from build123d import *

# Parameters (mm, degrees)
F0_W     = 57.15
F0_H     = 31.75
F1_DEPTH = 25.4
F3_DEPTH = 25.4


with BuildPart() as f1:
    # F0 (on Front) → F1 (new body)
    with BuildSketch(Plane.XZ):
        with Locations((28.575, 15.875)):
            Rectangle(F0_W, F0_H)
    extrude(amount=F1_DEPTH)

    # F2 (on face) → F3 (cut)
    with BuildSketch(Plane.XZ.offset(25.4)):
        with BuildLine():
            Line((57.15, 31.75), (38.1, 31.75))
            ThreePointArc((38.1, 31.75), (43.6796158184, 18.2796158184), (57.15, 12.7))
            Line((57.15, 12.7), (57.15, 31.75))
        make_face()
        with BuildLine():
            ThreePointArc((0, 25.4), (2.5236444149, 29.2263555851), (6.35, 31.75))
            Line((6.35, 31.75), (0, 31.75))
            Line((0, 31.75), (0, 25.4))
        make_face()
    extrude(amount=-F3_DEPTH, mode=Mode.SUBTRACT)


solid = f1.part
Geometry check sheet. Reference: the model listing, model coordinates, mm. Round coordinates to 2 decimals unless told otherwise and drop trailing zeros. Order: outer loops, then holes, each group sorted by start corner. A loop starts at its lowest first (then second) coordinate and runs counter-clockwise, first axis right, second up. Notation, with made-up numbers: M 70.5,-37.75 L 82.5,-37.75 A17 ccw 82.5,-23.75 Z; hole C -34,-0.75 d4. An arc over 180 degrees is marked long. Answer in a Markdown table with one row per item. Add a question column.
Item 1: Sectioned sample at A-A, the plane y = -23.5. Enter the section's corners in (x, z).
Item 2: Sectioned sample at C-C, the plane z = 15. Enter the section's corners in (x, y), plus the area to 3 significant figures.
Item 3: Material ranges on L1, parallel to X at y = -6.25, z = 25; L2, parallel to X at y = -4, z = 28; L3, parallel to Z at x = 5, y = -15.5, recorded low to high. Write a range as [from, to].
Item 4: Sectioned sample at B-B, the plane x = 41.5. Enter the section's corners in (y, z), plus the area to 3 significant figures.
Item 5: Depth check by flat-ended pin: pin 1 Ø8 at (x, y) = (27, -14) entering from -Z. Enter the tip coordinate at first touch or a pass-through.
Filled in:
| question | item | result |
|---|---|---|
| 1 | outline | M 0,0 L 57.15,0 L 57.15,12.7 A19.05 cw 38.1,31.75 L 6.35,31.75 A11.4 ccw 0,25.4 Z |
| 2 | outline | M 0,-25.4 L 48.08,-25.4 L 48.08,0 L 0,0 Z |
| 2 | area | 1,220 mm² |
| 3 | L1 | x = [0, 39.34] |
| 3 | L2 | x = [1.46, 38.47] |
| 3 | L3 | z = [0, 31.1] |
| 4 | outline | M -25.4,0 L 0,0 L 0,20.89 L -25.4,20.89 Z |
| 4 | area | 531 mm² |
| 5 | pin 1 | stops at z = 0 |
